```python
from build123d import *

# Parameters (mm, degrees)
BOSS_EXTRUDE2_DEPTH = 3


with BuildPart() as part:
    # Sketch6 → Boss-Extrude2 (new body)
    with BuildSketch(Plane(origin=(0, 0, -3), x_dir=(-1, 0, 0), z_dir=(0, 0, -1))):
        with BuildLine():
            Line((-19.25, 3.741713812), (0, -0.35))
            add(Edge.make_bspline(
                [(0, -0.35), (3.178862469, 6.495343287), (8.987756305, 8.032168144), (22.140633739, 13.071207305), (43.250433247, 17.69324185), (66.39602757, 18.219905629)],
                knots=[0, 0, 0, 0, 0, 0, 1, 1, 1, 1, 1, 1], degree=5))
            add(Edge.make_bspline(
                [(66.39602757, 18.219905629), (73.079858249, 18.217137873), (79.768873399, 18.101745103), (86.45, 17.815976098)],
                knots=[0.875945967, 0.875945967, 0.875945967, 0.875945967, 0.985673704, 0.985673704, 0.985673704, 0.985673704], degree=3))
            Line((86.45, 17.815976098), (86.45, 24.670250599))
            Line((86.45, 24.670250599), (89.45, 24.670250599))
            Line((89.45, 24.670250599), (89.45, 17.675984992))
            add(Edge.make_bspline(
                [(89.45, 17.675984992), (90.320899947, 17.631898595), (91.191632468, 17.584767892), (92.062168571, 17.534464817)],
                knots=[1.002100386, 1.002100386, 1.002100386, 1.002100386, 1.01640933, 1.01640933, 1.01640933, 1.01640933], degree=3))
            add(Edge.make_bspline(
                [(92.062168571, 17.534464817), (95.665977641, 17.334138157), (108.464938821, 16.428798519), (140.620964858, 12.117510077), (188.11962528, 1.017487261), (227.440155367, -4.385412225), (246.547152618, -10.292650589)],
                knots=[0, 0, 0, 0, 0.05922822, 0.210539222, 0.531730365, 0.859536637, 0.859536637, 0.859536637, 0.859536637], degree=3))
            add(Edge.make_bspline(
                [(246.547152618, -10.292650589), (248.808777451, -9.863624592), (247.588252624, -6.363600679), (247.543685046, -4.960441529)],
                knots=[0, 0, 0, 0, 1, 1, 1, 1], degree=3))
            add(Edge.make_bspline(
                [(247.543685046, -4.960441529), (248.441640739, -5.14429555), (249.235236144, -5.197240659)],
                knots=[0, 0, 0, 0.116478493, 0.116478493, 0.116478493], degree=2))
            add(Edge.make_bspline(
                [(249.235236144, -5.197240659), (255.254876243, -5.598843915), (255.27, 1.531581744)],
                knots=[0.116478493, 0.116478493, 0.116478493, 1, 1, 1], degree=2))
            Line((255.27, 1.531581744), (255.27, 58.507349411))
            Line((255.27, 58.507349411), (174.85, 63.193699149))
            Line((174.85, 63.193699149), (174.85, 58.185216861))
            Line((174.85, 58.185216861), (159.85, 59.059318403))
            Line((159.85, 59.059318403), (159.85, 64.067800692))
            Line((159.85, 64.067800692), (118.95, 66.451184232))
            Line((118.95, 66.451184232), (118.95, 61.943550172))
            Line((118.95, 61.943550172), (104.95, 62.759378279))
            Line((104.95, 62.759378279), (104.95, 67.267012338))
            Line((104.95, 67.267012338), (89.45, 68.170250599))
            Line((89.45, 68.170250599), (89.45, 62.370250599))
            Line((89.45, 62.370250599), (86.45, 62.370250599))
            Line((86.45, 62.370250599), (86.45, 68.043292799))
            Line((86.45, 68.043292799), (-16.333378442, 66.994986377))
            Line((-16.333378442, 66.994986377), (-19.25, 66.904044127))
            Line((-19.25, 66.904044127), (-19.25, 60.904044127))
            Line((-19.25, 60.904044127), (-22.25, 60.904044127))
            Line((-22.25, 60.904044127), (-22.25, 66.810502081))
            Line((-22.25, 66.810502081), (-111.531056313, 64.026657849))
            Line((-111.531056313, 64.026657849), (-111.531056313, 23.356657849))
            Line((-111.531056313, 23.356657849), (-22.25, 4.379383497))
            Line((-22.25, 4.379383497), (-22.25, 9.741713812))
            Line((-22.25, 9.741713812), (-19.25, 9.741713812))
            Line((-19.25, 9.741713812), (-19.25, 3.741713812))
        make_face()
        Polygon((-84.1, 54.203030213), (-26.1, 57.75847956), (-26.1, 17.874749636), (-84.1, 30.203030213), align=None, mode=Mode.SUBTRACT)
        with BuildLine():
            Line((-10.5, 21.65), (-10.5, 55.95))
            Line((-10.5, 55.95), (87.47, 56.949213898))
            Line((87.47, 56.949213898), (87.47, 30.129694509))
            ThreePointArc((87.47, 30.129694509), (86.67270256, 28.299174366), (84.789356805, 27.636229443))
            add(Edge.make_bspline(
                [(14.701665666, 21.959575817), (21.19900444, 24.808951329), (34.471850374, 27.925627057), (54.295468051, 29.219545771), (70.832055402, 28.62299092), (81.026620283, 27.908827105), (84.789356805, 27.636229443)],
                knots=[0.099500985, 0.099500985, 0.099500985, 0.099500985, 0.360279093, 0.592189537, 0.828480504, 0.96707438, 0.96707438, 0.96707438, 0.96707438], degree=3))
            Line((14.701665666, 21.959575817), (7.522354632, 18.142268428))
            Line((7.522354632, 18.142268428), (0, 21.65))
            Line((0, 21.65), (0, 16.35))
            Line((0, 16.35), (-3, 16.35))
            Line((-3, 16.35), (-3, 21.65))
            Line((-3, 21.65), (-10.5, 21.65))
        make_face(mode=Mode.SUBTRACT)
        Polygon((93.97, 30.170250599), (93.97, 55.670250599), (239.97, 45.483901662), (239.97, 9.104044127), (220.823057098, 7.643571), (170.32923345, 17.7710139), align=None, mode=Mode.SUBTRACT)
    extrude(amount=BOSS_EXTRUDE2_DEPTH)


solid = part.part
```
Part model, mm, in its own coordinate system. A direction names the side the tool comes from. Round coordinates to 2 decimals unless told otherwise and drop trailing zeros. Write each loop counter-clockwise with the first axis right and the second up, starting at its lowest first coordinate (ties: lowest second). Pieces come first, ordered by that corner, then holes. Notation, with made-up numbers: M 29,-30.5 L 65,-30.5 A28 ccw 65,-6.5 Z; hole C -35,-8 d3. An arc over 180 degrees is marked long. One line per question, with ' | ' between items.
(1) Probe line 1 along X through (y, z) = (33, -3.15); line 2 along Y through (x, z) = (-10, -5.4); line 3 along Y through (x, z) = (66, -4.1). List the from-to ranges inside material, lowest first.
Answer key:
line 1: x = -255.27 to -239.97, -93.97 to -87.47, 10.5 to 26.1, 84.1 to 111.53 | line 2: y = 7.82 to 19.46, 56.16 to 67.26 | line 3: y = 13.68 to 26.36, 55.31 to 65.45
(2) 3-axis set-ups, long thin cutter, end or side, ignore diameter. For faces 4 (the face through (-69, 21, -6)), 5 (the face through (-195.93, 12.636, -4.479)): which of +Z, -Z, +X, -X, +Y, -Y reach the whole face in a straight line?
Answer key:
face 4: -Z, +X, -X, +Y, -Y | face 5: +Z, -Z
(3) Saw through at B-B on x = 53. Write the cut outline in (y, z).
Answer key:
outline: M 10.92,-6 L 23.59,-6 L 23.59,-3 L 10.92,-3 Z; M 56.11,-6 L 65.85,-6 L 65.85,-3 L 56.11,-3 Z
(4) Two-plate mould, pull along Y, no slides. Class faces 1 (the face through (-69, 21, -3)), 2 (the face through (67.52, 14, -4.48)), 3 (the face through (54.69, 23.95, -4.48)): released by +Y, released by -Y, zero draft, split by the parting line, or undercut.
Answer key:
face 1: zero draft | face 2: released by -Y | face 3: undercut
(5) Saw through at C-C on y = 49. Write the cut outline in (x, z).
Answer key:
outline: M -255.27,-6 L -189.57,-6 L -189.57,-3 L -255.27,-3 Z; M -93.97,-6 L -87.47,-6 L -87.47,-3 L -93.97,-3 Z; M 10.5,-6 L 26.1,-6 L 26.1,-3 L 10.5,-3 Z; M 84.1,-6 L 111.53,-6 L 111.53,-3 L 84.1,-3 Z
(6) Saw through at D-D on z = -5.35. Count the separate pieces of the cut face and the enclosed holes in it, then the cut area to 3 significant figures.
Answer key:
separate pieces: 1 | enclosed holes: 3 | area: 10,600 mm^2
(7) Pin check, flat tips, straight feed: pin 1 (0.9 mm diameter, centred on x = 1, z = -4.5, fed in from +Y); pin 2 (12 mm diameter, centred on x = -103.5, y = 13.5, fed in from -Z); pin 3 (1 mm diameter, centred on x = -98.5, z = -4, fed in from +Y). Stop position of each tip, or through.
Answer key:
pin 1: stops at y = 67.16 | pin 2: stops at z = -6 | pin 3: stops at y = 67.67
(8) Saw through at A-A on y = 33.5. Write the cut outline in (x, z).
Answer key:
outline: M -255.27,-6 L -239.97,-6 L -239.97,-3 L -255.27,-3 Z; M -93.97,-6 L -87.47,-6 L -87.47,-3 L -93.97,-3 Z; M 10.5,-6 L 26.1,-6 L 26.1,-3 L 10.5,-3 Z; M 84.1,-6 L 111.53,-6 L 111.53,-3 L 84.1,-3 Z
